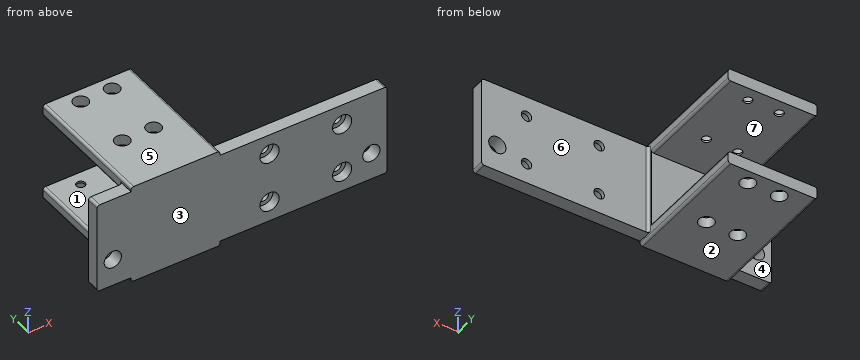
```python
from build123d import *

# Parameters (mm, degrees)
SKETCH1_W                                      = 105
SKETCH1_H                                      = 35
BOSS_EXTRUDE1_DEPTH                            = 5
SKETCH4_W                                      = 33.2
SKETCH4_H                                      = 35
BOSS_EXTRUDE2_DEPTH                            = 1.45
BOSS_EXTRUDE3_DEPTH                            = 17
CBORE_FOR_M2_5_SHCS1_AT_2_COUNT                = 2
CBORE_FOR_M2_5_SHCS1_AT_2_PITCH                = 12
CBORE_FOR_M2_5_SHCS1_AT_3_COUNT                = 2
CBORE_FOR_M2_5_SHCS1_AT_3_PITCH                = 24
CBORE_FOR_M2_5_SHCS1_AT_4_COUNT                = 2
CBORE_FOR_M2_5_SHCS1_AT_4_PITCH                = 26.83281573
BOSS_EXTRUDE5_DEPTH                            = 0.4
BOSS_EXTRUDE6_DEPTH                            = 0.4
CBORE_FOR_6_SOCKET_HEAD_CAP_SCREW1_D           = 3.997300108
CBORE_FOR_6_SOCKET_HEAD_CAP_SCREW1_CBORE_D     = 7.345020108
CBORE_FOR_6_SOCKET_HEAD_CAP_SCREW1_CBORE_DEPTH = 3.5052
SKETCH15_W                                     = 34
SKETCH15_H                                     = 44.5
CUT_EXTRUDE1_DEPTH                             = 14.5
SKETCH16_W                                     = 35
SKETCH16_H                                     = 5
BOSS_EXTRUDE7_DEPTH                            = 2
SKETCH17_W                                     = 35
SKETCH17_H                                     = 5
BOSS_EXTRUDE8_DEPTH                            = 4
M6_CLEARANCE_HOLE1_D                           = 6.6
FILLET1_R                                      = 1


with BuildPart() as part:
    # Sketch1 → Boss-Extrude1 (new body)
    with BuildSketch(Plane(origin=(0, 0, 0), x_dir=(1, 0, 0), z_dir=(0, 1, 0))):
        Rectangle(SKETCH1_W, SKETCH1_H)
    extrude(amount=BOSS_EXTRUDE1_DEPTH)

    # Sketch4 → Boss-Extrude2 (add)
    with BuildSketch(Plane(origin=(0, 5, 0), x_dir=(1, 0, 0), z_dir=(0, 1, 0))):
        with Locations((-24.5, 0)):
            Rectangle(SKETCH4_W, SKETCH4_H)
    extrude(amount=BOSS_EXTRUDE2_DEPTH)

    # Sketch5 → Boss-Extrude3 (add, symmetric)
    with BuildSketch(Plane.ZY.offset(24.5)):
        Polygon((-17.5, 0), (-19.25, 0), (-19.25, 50.95), (-14.25, 50.95), (-14.25, 6.45), (-17.5, 6.45), align=None)
    boss_extrude3 = extrude(amount=BOSS_EXTRUDE3_DEPTH, both=True)

    # Sketch9 → CBORE for M2.5 SHCS1 (revolve, cut)
    with BuildSketch(Plane(origin=(-30.5, 45.7, -19.25), x_dir=(0, 1, 0), z_dir=(1, 0, 0))):
        Polygon((0, 0), (0, 34.490420021), (1.65, 33.499), (1.65, 4), (2.85, 4), (2.85, 0), align=None)
    cbore_for_m2_5_shcs1 = revolve(axis=Axis((-30.5, 45.7, -25.6), (0, 0, 1)), mode=Mode.SUBTRACT)

    # CBORE for M2.5 SHCS1 at 2: CBORE for M2.5 SHCS1 ×2
    with Locations(*[(i * CBORE_FOR_M2_5_SHCS1_AT_2_PITCH, 0, 0) for i in range(1, CBORE_FOR_M2_5_SHCS1_AT_2_COUNT)]):
        add(cbore_for_m2_5_shcs1, mode=Mode.SUBTRACT)

    # CBORE for M2.5 SHCS1 at 3: CBORE for M2.5 SHCS1 ×2
    with Locations(*[(0, -i * CBORE_FOR_M2_5_SHCS1_AT_3_PITCH, 0) for i in range(1, CBORE_FOR_M2_5_SHCS1_AT_3_COUNT)]):
        add(cbore_for_m2_5_shcs1, mode=Mode.SUBTRACT)

    # CBORE for M2.5 SHCS1 at 4: CBORE for M2.5 SHCS1 ×2
    with Locations(*[Vector(0.44721359549995815, -0.8944271909999159, 0) * (i * CBORE_FOR_M2_5_SHCS1_AT_4_PITCH) for i in range(1, CBORE_FOR_M2_5_SHCS1_AT_4_COUNT)]):
        add(cbore_for_m2_5_shcs1, mode=Mode.SUBTRACT)

    # Mirror1: Boss-Extrude3, CBORE for M2.5 SHCS1 across plane
    add(boss_extrude3.mirror(Plane(origin=(0, 0, 0), x_dir=(1, 0, 0), z_dir=(0, 0, -1))))
    add(cbore_for_m2_5_shcs1.mirror(Plane(origin=(0, 0, 0), x_dir=(1, 0, 0), z_dir=(0, 0, -1))), mode=Mode.SUBTRACT)

    # Mirror1 copy 1 sketch → Mirror1 copy 1 (revolve, cut)
    with BuildSketch(Plane(origin=(-18.5, 45.7, 19.25), x_dir=(0, 1, 0), z_dir=(1, 0, 0))):
        Polygon((0, 0), (0, -34.490420021), (1.65, -33.499), (1.65, -4), (2.85, -4), (2.85, 0), align=None)
    revolve(axis=Axis((-18.5, 45.7, 25.6), (0, 0, 1)), mode=Mode.SUBTRACT)

    # Mirror1 copy 2 sketch → Mirror1 copy 2 (revolve, cut)
    with BuildSketch(Plane(origin=(-30.5, 21.7, 19.25), x_dir=(0, 1, 0), z_dir=(1, 0, 0))):
        Polygon((0, 0), (0, -34.490420021), (1.65, -33.499), (1.65, -4), (2.85, -4), (2.85, 0), align=None)
    revolve(axis=Axis((-30.5, 21.7, 25.6), (0, 0, 1)), mode=Mode.SUBTRACT)

    # Mirror1 copy 3 sketch → Mirror1 copy 3 (revolve, cut)
    with BuildSketch(Plane(origin=(-18.5, 21.7, 19.25), x_dir=(0, 1, 0), z_dir=(1, 0, 0))):
        Polygon((0, 0), (0, -34.490420021), (1.65, -33.499), (1.65, -4), (2.85, -4), (2.85, 0), align=None)
    revolve(axis=Axis((-18.5, 21.7, 25.6), (0, 0, 1)), mode=Mode.SUBTRACT)

    # Sketch11 → Boss-Extrude5 (add)
    with BuildSketch(Plane(origin=(-7.9, 0, 0), x_dir=(0, 0, -1), z_dir=(1, 0, 0))):
        Polygon((17.5, 5), (17.5, 6.45), (14.25, 6.45), (-14.25, 6.45), (-17.5, 6.45), (-17.5, 5), align=None)
    extrude(amount=BOSS_EXTRUDE5_DEPTH)

    # Sketch12 → Boss-Extrude6 (add)
    with BuildSketch(Plane.ZY.offset(41.1)):
        Polygon((17.5, 5), (17.5, 6.45), (14.25, 6.45), (-14.25, 6.45), (-17.5, 6.45), (-17.5, 5), align=None)
    extrude(amount=BOSS_EXTRUDE6_DEPTH)

    # CBORE for #6 Socket Head Cap Screw1 (through all)
    with Locations(Plane(origin=(0, 0, 0), x_dir=(-1, 0, 0), z_dir=(0, -1, 0))):
        with Locations((-39.325, 9.779), (-11.514, 9.779), (-39.325, -9.639687995), (-11.514, -9.779)):
            CounterBoreHole(CBORE_FOR_6_SOCKET_HEAD_CAP_SCREW1_D / 2, CBORE_FOR_6_SOCKET_HEAD_CAP_SCREW1_CBORE_D / 2, CBORE_FOR_6_SOCKET_HEAD_CAP_SCREW1_CBORE_DEPTH)

    # Sketch15 → Cut-Extrude1 (cut, symmetric)
    with BuildSketch(Plane(origin=(0, 0, 0), x_dir=(-1, 0, 0), z_dir=(0, 0, -1))):
        with Locations((24.5, 28.7)):
            Rectangle(SKETCH15_W, SKETCH15_H)
    extrude(amount=CUT_EXTRUDE1_DEPTH, both=True, mode=Mode.SUBTRACT)

    # Sketch16 → Boss-Extrude7 (add)
    with BuildSketch(Plane.ZY.offset(52.5)):
        with Locations((0, 2.5)):
            Rectangle(SKETCH16_W, SKETCH16_H)
    extrude(amount=BOSS_EXTRUDE7_DEPTH)

    # Sketch17 → Boss-Extrude8 (add)
    with BuildSketch(Plane(origin=(52.5, 0, 0), x_dir=(0, 0, -1), z_dir=(1, 0, 0))):
        with Locations((0, 2.5)):
            Rectangle(SKETCH17_W, SKETCH17_H)
    extrude(amount=BOSS_EXTRUDE8_DEPTH)

    # M6 Clearance Hole1 (through all)
    with Locations(Plane(origin=(0, 5, 0), x_dir=(1, 0, 0), z_dir=(0, 1, 0))):
        with Locations((-48.5, 7), (50.5, 7)):
            Hole(M6_CLEARANCE_HOLE1_D / 2)

    # Fillet1
    fillet1_edges = [part.edges().sort_by_distance(p)[0] for p in [
        (-7.5, 5, 0),
        (-41.5, 5, 0),
        (-7.5, 28.7, -14.5),
        (-41.5, 28.7, -14.5),
        (-7.5, 28.7, 14.5),
        (-41.5, 28.7, 14.5),
        (-54.5, 2.5, -17.5),
        (-54.5, 2.5, 17.5),
        (56.5, 2.5, 17.5),
        (56.5, 2.5, -17.5),
        (-41.5, 25.475, -19.25),
        (-7.5, 25.475, -19.25),
        (-41.5, 25.475, 19.25),
        (-7.5, 25.475, 19.25),
    ]]
    fillet(fillet1_edges, radius=FILLET1_R)


solid = part.part
```
Geometry: final body of the model. Coordinates: model frame, mm. Face numbers are marked on the shaded views. A direction names the side the tool comes from. Coordinates: 2 decimals unless noted, no trailing zeros. Order: outer loops, then holes, each group sorted by start corner. A loop starts at its lowest first (then second) coordinate and runs counter-clockwise, first axis right, second up. Notation, with made-up numbers: (50, 74.25) -> (74, 74.25) arc R34 ccw to (74, 109.25) -> close; hole circle Ø1 at (55.5, -10). An arc over 180 degrees is marked (long way). Write each question's results on one line, items separated by ' | '. Start each with the question number.
1) Set-up query: the marked faces 4, 5, 6 and 7. Return all of +Z, -Z, +X, -X, +Y, -Y with unobstructed straight access to the full face (end or side cutting, diameter ignored); none if empty.
2) Cut plane B-B, the plane y = 12. Output: boundary loops of the cut face in (x, z).
3) Material intervals for line 1 along X through (y, z) = (45.7, -18.1); line 2 along Y through (x, z) = (-30.5, -14.8); line 3 along Z through (x, y) = (50.5, 3.95), sorted ascending.
4) First-contact query: pin 1 (8 mm diameter, centred on y = 38, z = -15, fed in from -X); pin 2 (4.5 mm diameter, centred on x = -30.5, y = 21.7, fed in from -Z); pin 3 (1 mm diameter, centred on y = 13, z = 15, fed in from +X). Flat tips, straight axial feed; report the tip coordinate or a pass-through.
5) Cut plane D-D, the plane x = -18.5. State how many separate pieces and enclosed holes the cut face has, and give its area (3 significant figures).
6) Cut plane C-C, the plane z = -5. Output: boundary loops of the cut face in (x, y), and give its area (3 significant figures).
7) Cut plane A-A, the plane x = 50.5. Output: boundary loops of the cut face in (y, z).
8) Mould query, pull axis Z, two halves, no side actions, for the marked faces 1, 2 and 3. Classes: released by +Z, released by -Z, zero draft, split by the parting line, or undercut.
Checks:
1) face 4: +Z, -Z, -X, +Y | face 5: +Z, +X, -X, +Y, -Y | face 6: +Z, -Z, +X, +Y | face 7: +X, -X, +Y
2) outline: (-41.5, -18.25) arc R1 ccw to (-40.5, -19.25) -> (-8.5, -19.25) arc R1 ccw to (-7.5, -18.25) -> (-7.5, -15.5) arc R1 ccw to (-8.5, -14.5) -> (-40.5, -14.5) arc R1 ccw to (-41.5, -15.5) -> close; (-41.5, 15.5) arc R1 ccw to (-40.5, 14.5) -> (-8.5, 14.5) arc R1 ccw to (-7.5, 15.5) -> (-7.5, 18.25) arc R1 ccw to (-8.5, 19.25) -> (-40.5, 19.25) arc R1 ccw to (-41.5, 18.25) -> close
3) line 1: -41.5 to -33.35, -27.65 to -21.35, -15.65 to -7.5 | line 2: 0 to 20.05, 23.35 to 44.05, 47.35 to 50.95 | line 3: -17.5 to -10.3, -3.7 to 17.5
4) pin 1: x = -41.5 | pin 2: z = -15.25 | pin 3: x = -7.5
5) separate pieces: 5 | enclosed holes: 0 | area: 570 mm^2
6) outline: (-54.5, 0) -> (-51.12, 0) -> (-51.12, 5) -> (-54.5, 5) -> close; (-45.88, 0) -> (47.88, 0) -> (47.88, 5) -> (-6.5, 5) arc R1 cw to (-7.5, 6) -> (-7.5, 6.45) -> (-41.5, 6.45) -> (-41.5, 6) arc R1 cw to (-42.5, 5) -> (-45.88, 5) -> close; (53.12, 0) -> (56.5, 0) -> (56.5, 5) -> (53.12, 5) -> close | area: 552 mm^2
7) outline: (0, -17.5) -> (5, -17.5) -> (5, -10.3) -> (0, -10.3) -> close; (0, -3.7) -> (5, -3.7) -> (5, 17.5) -> (0, 17.5) -> close
8) face 1: undercut | face 2: released by -Z | face 3: zero draft
